```python
from build123d import *

# Parameters (mm, degrees)
F0_R     = 14.2875
F1_DEPTH = 25.4


with BuildPart() as f1:
    # F0 (on Front) → F1 (new body)
    with BuildSketch(Plane.XZ):
        with BuildLine():
            Line((9.5121844836, 26.9452959039), (0, 28.575))
            ThreePointArc((0, 28.575), (-28.575, 0), (0, -28.575))
            Line((0, -28.575), (9.5121844836, -26.9452959039))
            ThreePointArc((9.5121844836, -26.9452959039), (23.3274655355, -16.5033322905), (28.575, 0))
            ThreePointArc((28.575, 0), (23.3274655355, 16.5033322905), (9.5121844836, 26.9452959039))
        make_face()
        with BuildLine():
            ThreePointArc((-13.4703841816, 4.7625), (0, 14.2875), (13.4703841816, 4.7625))
            Line((13.4703841816, 4.7625), (19.05, 4.7625))
            Line((19.05, 4.7625), (19.05, -4.7625))
            Line((19.05, -4.7625), (13.4703841816, -4.7625))
            ThreePointArc((13.4703841816, -4.7625), (0, -14.2875), (-13.4703841816, -4.7625))
            Line((-13.4703841816, -4.7625), (-19.05, -4.7625))
            Line((-19.05, -4.7625), (-19.05, 4.7625))
            Line((-19.05, 4.7625), (-13.4703841816, 4.7625))
        make_face(mode=Mode.SUBTRACT)
        with BuildLine():
            Line((57.1919272622, 18.7764181619), (9.5121844836, 26.9452959039))
            ThreePointArc((9.5121844836, 26.9452959039), (23.3274655355, 16.5033322905), (28.575, 0))
            ThreePointArc((28.575, 0), (23.3274655355, -16.5033322905), (9.5121844836, -26.9452959039))
            Line((9.5121844836, -26.9452959039), (57.1919272622, -18.7764181619))
            ThreePointArc((57.1919272622, -18.7764181619), (34.925, 0), (57.1919272622, 18.7764181619))
        make_face()
        with BuildLine():
            ThreePointArc((73.025, 0), (68.5383952831, 12.2804730295), (57.1919272622, 18.7764181619))
            ThreePointArc((57.1919272622, 18.7764181619), (34.925, 0), (57.1919272622, -18.7764181619))
            ThreePointArc((57.1919272622, -18.7764181619), (68.5383952831, -12.2804730295), (73.025, 0))
        make_face()
        with Locations((53.975, 0)):
            Circle(F0_R, mode=Mode.SUBTRACT)
        with BuildLine():
            ThreePointArc((-13.4703841816, -4.7625), (-14.2875, 0), (-13.4703841816, 4.7625))
            Line((-13.4703841816, 4.7625), (-19.05, 4.7625))
            Line((-19.05, 4.7625), (-19.05, -4.7625))
            Line((-19.05, -4.7625), (-13.4703841816, -4.7625))
        make_face()
    extrude(amount=F1_DEPTH)


solid = f1.part
```
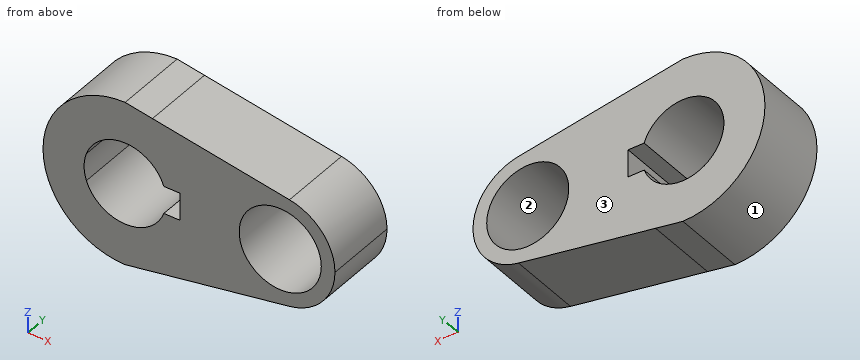
Input: part model. Units: mm. Frame: model coordinates. Face numbers are marked on the shaded views. Coordinates: 2 decimals unless noted, no trailing zeros. Write each loop counter-clockwise with the first axis right and the second up, starting at its lowest first coordinate (ties: lowest second). Pieces come first, ordered by that corner, then holes. Notation, with made-up numbers: (23.25, -0.75) -> (71.25, -0.75) arc R6 ccw to (71.25, 4.25) -> close; hole circle Ø9 at (5, 19.5). An arc over 180 degrees is marked (long way). Write each question's results on one line, items separated by ' | '.
Item 1: Section query A-A on y = -21.75. Count the separate pieces of the cut face and the enclosed holes in it, plus the area to 3 significant figures.
Conclusion:
separate pieces: 1 | enclosed holes: 2 | area: 3,110 mm^2
Item 2: Section query B-B on x = 47. Return loops of the section in (y, z).
Conclusion:
outline: (-25.4, -20.52) -> (0, -20.52) -> (0, -12.47) -> (-25.4, -12.47) -> close; (-25.4, 12.47) -> (0, 12.47) -> (0, 20.52) -> (-25.4, 20.52) -> close
Item 3: Section query D-D on x = 64. Return loops of the section in (y, z), plus the area to 3 significant figures.
Conclusion:
outline: (-25.4, -16.2) -> (0, -16.2) -> (0, -10.18) -> (-25.4, -10.18) -> close; (-25.4, 10.18) -> (0, 10.18) -> (0, 16.2) -> (-25.4, 16.2) -> close | area: 306 mm^2
Item 4: Material intervals for probe 1 along X at (y, z) = (-5.75, -5); probe 2 along X at (y, z) = (-12.5, 8); probe 3 along Z at (x, y) = (12, -16.75), sorted ascending.
Conclusion:
probe 1: x = -28.13 to -13.38, 13.38 to 40.59, 67.36 to 72.36 | probe 2: x = -27.43 to -11.84, 11.84 to 42.14, 65.81 to 71.26 | probe 3: z = -26.52 to -7.75, 7.75 to 26.52
Item 5: Section query C-C on z = -11.5. Return loops of the section in (x, y), plus the area to 3 significant figures.
Conclusion:
outline: (-26.16, -25.4) -> (-8.48, -25.4) -> (-8.48, 0) -> (-26.16, 0) -> close; (8.48, -25.4) -> (45.5, -25.4) -> (45.5, 0) -> (8.48, 0) -> close; (62.45, -25.4) -> (69.16, -25.4) -> (69.16, 0) -> (62.45, 0) -> close | area: 1,560 mm^2
Item 6: Mould query, pull axis Z, two halves, no side actions, for the marked faces 1, 2 and 3. Classes: +Z half, -Z half, draft (parallel to the pull), parting line (faces both ways), or undercut.
Conclusion:
face 1: parting line | face 2: undercut | face 3: draft
Item 7: Pin query (flat end, axial travel): pin 1 Ø6 at (x, y) = (15, -11.5) entering from +Z; pin 2 Ø5 at (x, y) = (-5.5, -12.5) entering from -Z; pin 3 Ø6 at (x, y) = (6.5, -8) entering from +Z; pin 4 Ø12 at (x, z) = (49.5, 0.5) entering from +Y. Return the tip coordinate at first contact, or that it passes through.
Conclusion:
pin 1: stops at z = 26.52 | pin 2: stops at z = -28.42 | pin 3: stops at z = 27.98 | pin 4: passes through
